from build123d import *

# Parameters (mm, degrees)
SKETCH1_R                = 13.97
SKETCH1_R_2              = 1.275
BOSS_EXTRUDE1_DEPTH      = 3.048
BOSS_EXTRUDE2_DEPTH      = 7.62
BOSS_EXTRUDE2_DEPTH_BACK = 3.048
SKETCH2_R                = 7.62
SKETCH2_R_2              = 1.275
CUT_EXTRUDE2_DEPTH       = 107.252483849
SKETCH6_R                = 8.89
SKETCH6_R_2              = 3.937
BOSS_EXTRUDE3_DEPTH      = 4.572
FILLET2_R                = 3.048
SKETCH8_W                = 176.271388165
SKETCH8_H                = 26.360341331
CUT_EXTRUDE3_DEPTH       = 107.252483849


with BuildPart() as part:
    # Sketch1 → Boss-Extrude1 (new body)
    with BuildSketch(Plane(origin=(0, 0, 0), x_dir=(1, 0, 0), z_dir=(0, 1, 0))):
        with Locations(Location((0, 0, 0), (0, 0, 90))):
            Circle(SKETCH1_R)
        with Locations(Location((0, 9.5, 0), (0, 0, 90))):
            Circle(SKETCH1_R_2, mode=Mode.SUBTRACT)
        with Locations(Location((9.5, 0, 0), (0, 0, 90))):
            Circle(SKETCH1_R_2, mode=Mode.SUBTRACT)
        with Locations(Location((0, -9.5, 0), (0, 0, 90))):
            Circle(SKETCH1_R_2, mode=Mode.SUBTRACT)
        with Locations(Location((-9.5, 0, 0), (0, 0, 90))):
            Circle(SKETCH1_R_2, mode=Mode.SUBTRACT)
    extrude(amount=BOSS_EXTRUDE1_DEPTH)

    # Sketch2 → Boss-Extrude2 (add, two sides: drawn at the far end of the back side and taken through both)
    with BuildSketch(Plane(origin=(0, 3.048, 0), x_dir=(1, 0, 0), z_dir=(0, 1, 0)).offset(-BOSS_EXTRUDE2_DEPTH_BACK)):
        with BuildLine():
            Line((-96.52, -14.605), (96.52, -14.605))
            ThreePointArc((96.52, -14.605), (100.112102448, -13.117102448), (101.6, -9.525))
            Line((101.6, -9.525), (101.6, 9.525))
            ThreePointArc((101.6, 9.525), (100.112102448, 13.117102448), (96.52, 14.605))
            Line((96.52, 14.605), (-96.52, 14.605))
            ThreePointArc((-96.52, 14.605), (-100.112102448, 13.117102448), (-101.6, 9.525))
            Line((-101.6, 9.525), (-101.6, -9.525))
            ThreePointArc((-101.6, -9.525), (-100.112102448, -13.117102448), (-96.52, -14.605))
        make_face()
        with Locations(Location((-88.9, 0, 0), (0, 0, 270))):
            Circle(SKETCH2_R, mode=Mode.SUBTRACT)
        with Locations(Location((88.9, 0, 0), (0, 0, 270))):
            Circle(SKETCH2_R, mode=Mode.SUBTRACT)
        with Locations(Location((9.5, 0, 0), (0, 0, 90))):
            Circle(SKETCH2_R_2, mode=Mode.SUBTRACT)
        with Locations(Location((0, 9.5, 0), (0, 0, 90))):
            Circle(SKETCH2_R_2, mode=Mode.SUBTRACT)
        with Locations(Location((-9.5, 0, 0), (0, 0, 90))):
            Circle(SKETCH2_R_2, mode=Mode.SUBTRACT)
        with Locations(Location((0, -9.5, 0), (0, 0, 90))):
            Circle(SKETCH2_R_2, mode=Mode.SUBTRACT)
    extrude(amount=BOSS_EXTRUDE2_DEPTH + BOSS_EXTRUDE2_DEPTH_BACK)

    # Sketch5 → Cut-Extrude2 (cut, through all)
    with BuildSketch(Plane(origin=(0, 0, -14.605), x_dir=(-1, 0, 0), z_dir=(0, 0, -1))):
        Polygon((-76.2, 3.81), (0, 3.81), (76.2, 3.81), (76.2, 10.668), (-76.2, 10.668), align=None)
    extrude(amount=-CUT_EXTRUDE2_DEPTH, mode=Mode.SUBTRACT)

    # Sketch6 → Boss-Extrude3 (add)
    # profile 1 of 2: a face of its own
    with BuildSketch(Plane.XZ):
        with Locations((-88.9, 0)):
            Circle(SKETCH6_R)
        with Locations(Location((-88.9, 0, 0), (0, 0, 270))):
            Circle(SKETCH6_R_2, mode=Mode.SUBTRACT)
    # profile 2 of 2: a face of its own
    with BuildSketch(Plane.XZ):
        with Locations((88.9, 0)):
            Circle(SKETCH6_R)
        with Locations(Location((88.9, 0, 0), (0, 0, 270))):
            Circle(SKETCH6_R_2, mode=Mode.SUBTRACT)
    extrude(amount=-BOSS_EXTRUDE3_DEPTH)

    # Fillet2
    fillet2_edges = [part.edges().sort_by_distance(p)[0] for p in [
        (-76.2, 3.81, 0),
        (76.2, 3.81, 0),
    ]]
    fillet(fillet2_edges, radius=FILLET2_R)

    # Sketch8 → Cut-Extrude3 (cut, through all)
    with BuildSketch(Plane.XY.offset(14.605)):
        with Locations((19.448788421, -1.041773615)):
            Rectangle(SKETCH8_W, SKETCH8_H)
    extrude(amount=-CUT_EXTRUDE3_DEPTH, mode=Mode.SUBTRACT)


solid = part.part
Read the model definition and answer for the solid it produces. Units are mm, in the model's axes. A direction names the side the tool comes from. Coordinates: 2 decimals unless noted, no trailing zeros. Loops run counter-clockwise (first coordinate to the right, second up) from the corner with the lowest first, then second, coordinate; pieces in that order, holes last.
Q1. The part is cut by section A-A on z = 0. Write down the section's boundary in (x, y).
Q2. The part is cut by section B-B on x = -88.9. Write down the section's boundary in (y, z) (3 decimals), and give its area (3 significant figures).
Q3. Which of the six approach directions +Z, -Z, +X, -X, +Y, -Y give full straight-line access (tool end or side, diameter ignored) to faces 4 (the face through (-81, 10.668, 0)), 5 (the face through (-76.2, 9, 0)), 6 (the face through (-86, 4.572, -3))?
Q4. The part is cut by section C-C on y = 7.25. Write down the section's boundary in (x, z) (3 decimals).
Q5. The part is cut by section D-D on z = 6.5. Write down the section's boundary in (x, y).
Q6. Each of these flat-tipped pins is pushed along its axis until it touches: pin 1 Ø4 at (y, z) = (9.5, 1) entering from +X; pin 2 Ø7.5 at (x, z) = (-91.5, 0) entering from +Y; pin 3 Ø5 at (x, z) = (-71, -4.5) entering from +Y. Where does it stop, or does it pass through?
Q7. Consider probe 1 along X at (y, z) = (2.15, 0); probe 2 along X at (y, z) = (8.25, 0); probe 3 along Z at (x, y) = (-88.9, 8.5) (3 decimals). Determine where each line is inside the solid, lowest interval first.
Q8. The mould has two halves that part along Z. Classify faces 1 (the face through (-86, 5, -14.605)), 2 (the face through (-84.997, 2.254, 0.513)), 3 (the face through (-101.6, 5, 0)): +Z half, -Z half, draft (parallel to the pull), parting line (faces both ways), or undercut.
Results below:
1. outline: (-101.6, 0) - (-92.84, 0) - (-92.84, 4.57) - (-96.52, 4.57) - (-96.52, 10.67) - (-101.6, 10.67) - close; (-84.96, 0) - (-68.69, 0) - (-68.69, 3.81) - (-73.15, 3.81) arc R3.05 cw to (-76.2, 6.86) - (-76.2, 10.67) - (-81.28, 10.67) - (-81.28, 4.57) - (-84.96, 4.57) - close
2. outline: (0, -14.605) - (10.668, -14.605) - (10.668, -7.62) - (4.572, -7.62) - (4.572, -3.937) - (0, -3.937) - close; (0, 3.937) - (4.572, 3.937) - (4.572, 7.62) - (10.668, 7.62) - (10.668, 14.605) - (0, 14.605) - close
2. area: 183 mm2
3. face 4: +Z, -Z, +X, -X, +Y
3. face 5: +Z, -Z, +X, +Y
3. face 6: +Y
4. outline: (-101.6, -9.525) arc R5.08 ccw to (-96.52, -14.605) - (-76.2, -14.605) - (-76.2, 14.605) - (-96.52, 14.605) arc R5.08 ccw to (-101.6, 9.525) - close; hole circle Ø15.24 at (-88.9, 0)
5. outline: (-101.6, 0) - (-68.69, 0) - (-68.69, 3.81) - (-73.15, 3.81) arc R3.05 cw to (-76.2, 6.86) - (-76.2, 10.67) - (-84.92, 10.67) - (-84.92, 4.57) - (-92.88, 4.57) - (-92.88, 10.67) - (-101.6, 10.67) - close
6. pin 1: stops at x = -76.2
6. pin 2: stops at y = 4.57
6. pin 3: stops at y = 3.83
7. probe 1: x = -101.6 to -92.84, -84.96 to -68.69
7. probe 2: x = -101.6 to -96.52, -81.28 to -76.2
7. probe 3: z = -14.605 to -7.62, 7.62 to 14.605
8. face 1: -Z half
8. face 2: undercut
8. face 3: draft
